from build123d import *

# Parameters (mm, degrees)
SKETCH1_W           = 52
SKETCH1_H           = 25
SKETCH1_W_2         = 2
BOSS_EXTRUDE1_DEPTH = 2
SKETCH1_3_W         = 2
SKETCH1_3_H         = 25
BOSS_EXTRUDE2_DEPTH = 65
FILLET4_R           = 2
SKETCH2_R           = 1.5
SKETCH2_R_2         = 4
CUT_EXTRUDE1_DEPTH  = 65
SKETCH3_R           = 4
SKETCH3_R_2         = 1.5
CUT_EXTRUDE2_DEPTH  = 65


with BuildPart() as part:
    # Sketch1 → Boss-Extrude1 (new body)
    with BuildSketch(Plane(origin=(0, 0, 0), x_dir=(1, 0, 0), z_dir=(0, 1, 0))):
        Rectangle(SKETCH1_W, SKETCH1_H)
        with Locations((-27, 0)):
            Rectangle(SKETCH1_W_2, SKETCH1_H)
        with Locations((27, 0)):
            Rectangle(SKETCH1_W_2, SKETCH1_H)
    extrude(amount=-BOSS_EXTRUDE1_DEPTH)

    # Sketch1_3 → Boss-Extrude2 (add)
    with BuildSketch(Plane(origin=(0, 0, 0), x_dir=(1, 0, 0), z_dir=(0, 1, 0))):
        with Locations((-27, 0)):
            Rectangle(SKETCH1_3_W, SKETCH1_3_H)
        with Locations((27, 0)):
            Rectangle(SKETCH1_3_W, SKETCH1_3_H)
    extrude(amount=BOSS_EXTRUDE2_DEPTH)

    # Fillet4
    fillet4_edges = [part.edges().sort_by_distance(p)[0] for p in [
        (-28, -2, 0),
        (-26, 0, 0),
        (28, -2, 0),
        (26, 0, 0),
    ]]
    fillet(fillet4_edges, radius=FILLET4_R)

    # Sketch2 → Cut-Extrude1 (cut)
    with BuildSketch(Plane(origin=(28, 0, 0), x_dir=(0, 0, -1), z_dir=(1, 0, 0))):
        with BuildLine():
            Line((-12.5, 65), (-12.5, 52.5))
            ThreePointArc((-12.5, 52.5), (-8.838834765, 61.338834765), (0, 65))
            Line((0, 65), (-12.5, 65))
        make_face()
        with BuildLine():
            Line((12.5, 65), (0, 65))
            ThreePointArc((0, 65), (8.838834765, 61.338834765), (12.5, 52.5))
            Line((12.5, 52.5), (12.5, 65))
        make_face()
        with Locations((0, 31.5)):
            Circle(SKETCH2_R)
        with Locations((0, 14.5)):
            Circle(SKETCH2_R)
        with Locations((0, 50)):
            Circle(SKETCH2_R_2)
        with Locations((-7, 50)):
            Circle(SKETCH2_R)
        with Locations((0, 57)):
            Circle(SKETCH2_R)
        with Locations((7, 50)):
            Circle(SKETCH2_R)
        with Locations((0, 43)):
            Circle(SKETCH2_R)
    extrude(amount=-CUT_EXTRUDE1_DEPTH, mode=Mode.SUBTRACT)

    # Sketch3 → Cut-Extrude2 (cut)
    with BuildSketch(Plane(origin=(0, 0, 0), x_dir=(1, 0, 0), z_dir=(0, 1, 0))):
        Circle(SKETCH3_R)
        with Locations((0, 7)):
            Circle(SKETCH3_R_2)
        with Locations((7, 0)):
            Circle(SKETCH3_R_2)
        with Locations((0, -7)):
            Circle(SKETCH3_R_2)
        with Locations((-7, 0)):
            Circle(SKETCH3_R_2)
        with Locations((-18.5, 0)):
            Circle(SKETCH3_R_2)
        with Locations((18.5, 0)):
            Circle(SKETCH3_R_2)
    extrude(amount=-CUT_EXTRUDE2_DEPTH, mode=Mode.SUBTRACT)


solid = part.part
Source: CAD feature listing. Evaluate the final solid. Frame: model axes, mm. A direction names the side the tool comes from. Round coordinates to 2 decimals unless told otherwise and drop trailing zeros. Loops run counter-clockwise (first coordinate to the right, second up) from the corner with the lowest first, then second, coordinate; pieces in that order, holes last. Notation, with made-up numbers: (72.25, -39.5) -> (107.25, -39.5) arc R18 cw to (107.25, -29.5) -> close; hole circle Ø2 at (-2, 8.5). An arc over 180 degrees is marked (long way). Answer as a JSON object with one key per item and string values. Group by question number.
Q1. Access query for faces 4 (the flat face through (5, 0, 0)), 5 (the cylindrical face through (-0.867, -0.986, 3.905)). Directions: +Z, -Z, +X, -X, +Y, -Y. A direction counts if a zero-diameter tool reaches every point of the face in a straight line with its end or side. Return the directions, or none.
Q2. Section query C-C (x = 0). Output: boundary loops of the cut face in (y, z), plus the area to 3 significant figures.
Q3. Contact query for flat-ended pins moving along their axis: P1, Ø2.5, axis at y = 14.5, z = 0, coming from the +X side; P2, Ø3.5, axis at x = 0, z = -7, coming from the +Y side; P3, Ø10, axis at x = 19.5, z = -5, coming from the +Y side. Output: stop coordinate, or through.
Q4. Ray query, line 1 (Z direction, x = 0, y = -1.3); line 2 (X direction, y = 48.5, z = 8.5); line 3 (Y direction, x = 26.95, z = 0). Return the intervals inside material, ascending. Write a range as from..to.
Q5. Section query D-D (z = 3.25). Output: boundary loops of the cut face in (x, y), plus the area to 3 significant figures.
Q6. Mould query, pull axis X, two halves, no side actions, for faces 1 (the cylindrical face through (25.43, 0.6, -0.18)), 2 (the cylindrical face through (-27.43, -1.4, -0.18)), 3 (the cylindrical face through (27, 13, 0)). Classes: pulls with the +X half, pulls with the -X half, needs draft (parallel to the pull), parting line crosses it, or undercut.
Q7. Section query A-A (x = -7). Output: boundary loops of the cut face in (y, z), plus the area to 3 significant figures.
Q8. Section query B-B (y = 9). Output: boundary loops of the cut face in (x, z).
Completed:
{
 "1": {"face 4": "+Z, -Z, +Y", "face 5": "+Y, -Y"},
 "2": {"outline": "(-2, -12.5) -> (0, -12.5) -> (0, -8.5) -> (-2, -8.5) -> close; (-2, -5.5) -> (0, -5.5) -> (0, -4) -> (-2, -4) -> close; (-2, 4) -> (0, 4) -> (0, 5.5) -> (-2, 5.5) -> close; (-2, 8.5) -> (0, 8.5) -> (0, 12.5) -> (-2, 12.5) -> close", "area": "22.0 mm²"},
 "3": {"P1": "through", "P2": "y = 0", "P3": "y = 0.06"},
 "4": {"line 1": "-12.5..-8.5, -5.5..-4, 4..5.5, 8.5..12.5", "line 2": "-28..-26, 26..28", "line 3": "-1.76..13, 16..30, 33..41.5, 44.5..46, 54..55.5, 58.5..65"},
 "5": {"outline": "(-28, 0) arc R2 ccw to (-26, -2) -> (-2.33, -2) -> (-2.33, 0) -> (-24, 0) arc R2 cw to (-26, 2) -> (-26, 47.67) -> (-28, 47.67) -> close; (-28, 52.33) -> (-26, 52.33) -> (-26, 64.57) -> (-28, 64.57) -> close; (2.33, -2) -> (26, -2) arc R2 ccw to (28, 0) -> (28, 47.67) -> (26, 47.67) -> (26, 2) arc R2 cw to (24, 0) -> (2.33, 0) -> close; (26, 52.33) -> (28, 52.33) -> (28, 64.57) -> (26, 64.57) -> close", "area": "342 mm²"},
 "6": {"face 1": "undercut", "face 2": "pulls with the -X half", "face 3": "needs draft"},
 "7": {"outline": "(-2, -12.5) -> (0, -12.5) -> (0, -1.5) -> (-2, -1.5) -> close; (-2, 1.5) -> (0, 1.5) -> (0, 12.5) -> (-2, 12.5) -> close", "area": "44.0 mm²"},
 "8": {"outline": "(-28, -12.5) -> (-26, -12.5) -> (-26, 12.5) -> (-28, 12.5) -> close; (26, -12.5) -> (28, -12.5) -> (28, 12.5) -> (26, 12.5) -> close"}
}
